Geometry check sheet. Reference: the model listing, model coordinates, mm. Give positions to 0.01 mm unless a question says otherwise; leave off trailing zeros. Order: outer loops, then holes, each group sorted by start corner. A loop starts at its lowest first (then second) coordinate and runs counter-clockwise, first axis right, second up.
from build123d import *

# Parameters (mm, degrees)
CHAMFER1_SIZE           = 1.27
CUT_EXTRUDE1_DEPTH      = 769.402477547
CUT_EXTRUDE1_DEPTH_BACK = 769.402477547
SKETCH2_R               = 3.175


with BuildPart() as part:
    # Sketch1 → Revolve1 (revolve)
    with BuildSketch(Plane.XY, mode=Mode.PRIVATE) as revolve1_sk:
        Polygon((0, 0), (0, 768.35), (-6.35, 768.35), (-6.35, 12.7), (-4.7625, 12.7), (-4.7625, 0), align=None)
    revolve(revolve1_sk.sketch.rotate(Axis((0, 0, 0), (0, 1, 0)), 270), axis=Axis((0, 0, 0), (0, 1, 0)))

    # Chamfer1
    chamfer1_edges = [part.edges().sort_by_distance(p)[0] for p in [
        (0, 0, 4.7625),
    ]]
    chamfer(chamfer1_edges, length=CHAMFER1_SIZE)

    # Sketch2 → Cut-Extrude1 (cut, two sides: drawn at the far end of the back side and taken through both)
    with BuildSketch(Plane.XY.offset(-CUT_EXTRUDE1_DEPTH_BACK)):
        with Locations((0, 749.3)):
            Circle(SKETCH2_R)
    extrude(amount=CUT_EXTRUDE1_DEPTH + CUT_EXTRUDE1_DEPTH_BACK, mode=Mode.SUBTRACT)


solid = part.part
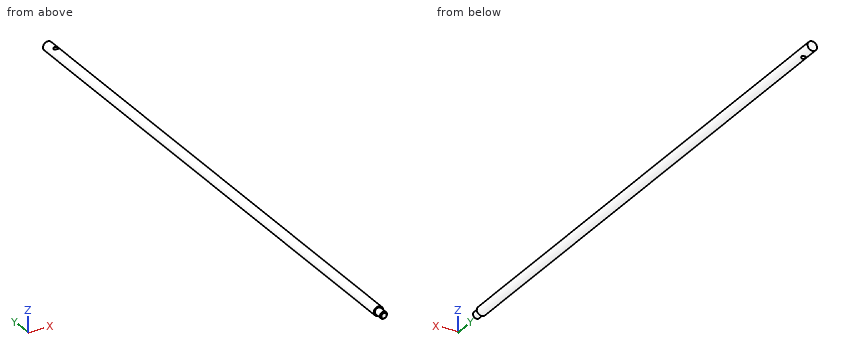
Item 1: Sectioned sample at A-A (y = 475). Enter the section's corners in (x, z).
Reported:
outline: circle Ø12.7 at (0, 0)
Item 2: Gauge pin test, flat ends, axial feed: pin 1 (3 mm diameter, centred on x = 3, y = 581, fed in from +Z); pin 2 (4 mm diameter, centred on x = 0, z = -3, fed in from -Y); pin 3 (1.5 mm diameter, centred on y = 659.5, z = -3.5, fed in from +X); pin 4 (5 mm diameter, centred on x = 3, y = 384, fed in from -Z). Record the tip position at first contact, or that the pin passes through.
Reported:
pin 1: stops at z = 6.17
pin 2: stops at y = 0
pin 3: stops at x = 5.72
pin 4: stops at z = -6.33
Item 3: Scan lines: L1, parallel to Y at x = 0, z = -0.25 (3 decimals); L2, parallel to X at y = 749.3, z = -1.25 (3 decimals); L3, parallel to Y at x = -4.5, z = 3.5. Record each from-to range of solid material in increasing order.
Reported:
L1: y = 0 to 746.125, 752.475 to 768.35
L2: x = -6.226 to -3.175, 3.175 to 6.226
L3: y = 12.7 to 768.35
